Geometry: final body of the model. Coordinates: model frame, mm. Face numbers are marked on the shaded views. A direction names the side the tool comes from. Give positions to 0.01 mm unless a question says otherwise; leave off trailing zeros. Write each loop counter-clockwise with the first axis right and the second up, starting at its lowest first coordinate (ties: lowest second). Pieces come first, ordered by that corner, then holes.
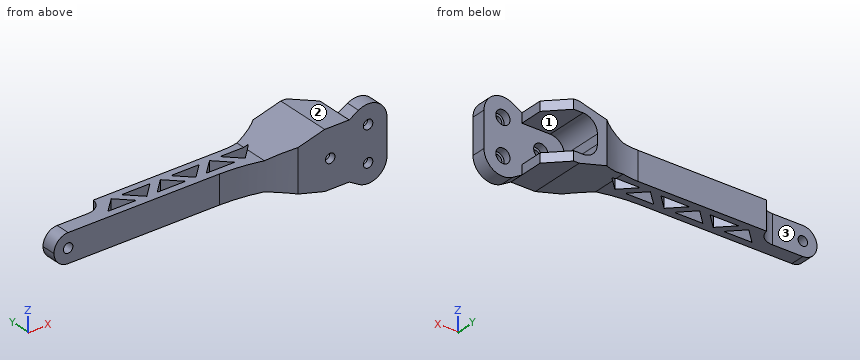
from build123d import *

# Parameters (mm, degrees)
BOSS_EXTRUDE1_DEPTH                     = 15
BOSS_EXTRUDE1_DEPTH_BACK                = 15
FILLET1_R                               = 15
BOSS_EXTRUDE2_DEPTH                     = 60
CUT_EXTRUDE5_DEPTH                      = 43
CUT_EXTRUDE5_DEPTH_BACK                 = 43
SKETCH1_6_OUTSIDE_W                     = 364.354
SKETCH1_6_OUTSIDE_H                     = 124.354
BOSS_EXTRUDE3_DEPTH                     = 15
CUT_EXTRUDE7_DEPTH                      = 256.415087263
CBORE_FOR_M5_HEX_HEAD_BOLT1_D           = 10
CBORE_FOR_M5_HEX_HEAD_BOLT1_DEPTH       = 20
CBORE_FOR_M5_HEX_HEAD_BOLT1_CBORE_D     = 15
CBORE_FOR_M5_HEX_HEAD_BOLT1_CBORE_DEPTH = 8
CBORE_FOR_M5_HEX_HEAD_BOLT1_TIP         = 3.004303095
F_10_0MM_DOWEL_HOLE1_D                  = 10
CUT_EXTRUDE9_DEPTH                      = 259.016066246
CUT_EXTRUDE14_DEPTH                     = 259.016066246


with BuildPart() as part:
    # Sketch1 → Boss-Extrude1 (new, two sides: drawn at the far end of the back side and taken through both)
    with BuildSketch(Plane.XY.offset(-BOSS_EXTRUDE1_DEPTH_BACK)):
        with BuildLine():
            Line((0, 0), (-91.545543809, 0))
            Line((-91.545543809, 0), (-91.545543809, 15))
            Line((-91.545543809, 15), (-44.293783158, 15))
            ThreePointArc((-44.293783158, 15), (-32.674833119, 19.252272915), (-26.545543809, 30))
            Line((-26.545543809, 30), (109.126292876, 30))
            ThreePointArc((109.126292876, 30), (132.446309196, 33.71762603), (153.454456191, 44.501950965))
            Line((153.454456191, 44.501950965), (188.454456191, 44.501950965))
            Line((188.454456191, 44.501950965), (208.454456191, 24.501950965))
            Line((208.454456191, 24.501950965), (208.454456191, 0))
            Line((208.454456191, 0), (208.454456191, -15.498049035))
            Line((208.454456191, -15.498049035), (154.553796185, -15.498049035))
            ThreePointArc((154.553796185, -15.498049035), (119.809900794, -3.919403897), (83.397793421, 0))
            Line((83.397793421, 0), (0, 0))
        make_face()
    extrude(amount=BOSS_EXTRUDE1_DEPTH + BOSS_EXTRUDE1_DEPTH_BACK)

    # Fillet1
    fillet1_edges = [part.edges().sort_by_distance(p)[0] for p in [
        (-91.545543809, 7.5, 15),
        (-91.545543809, 7.5, -15),
    ]]
    fillet(fillet1_edges, radius=FILLET1_R - 0.0001)  # a hair under: the kernel refuses the full size

    # Sketch2 → Boss-Extrude2 (add)
    with BuildSketch(Plane.XZ.offset(15.498049035)):
        Polygon((126.618755864, -15), (153.454456191, -22.190604231), (182.599517977, -30), (208.454456191, -30), (208.454456191, 30), (182.599517977, 30), (153.454456191, 22.190604231), (126.618755864, 15), align=None)
    extrude(amount=-BOSS_EXTRUDE2_DEPTH)

    # Sketch1<6> outside → Cut-Extrude5 (cut, two sides: drawn at the far end of the back side and taken through both)
    with BuildSketch(Plane.XY.offset(-CUT_EXTRUDE5_DEPTH_BACK)):
        with Locations((58.454, 14.502)):
            Rectangle(SKETCH1_6_OUTSIDE_W, SKETCH1_6_OUTSIDE_H)
        with BuildLine():
            Line((0, 0), (-91.545543809, 0))
            Line((-91.545543809, 0), (-91.545543809, 15))
            Line((-91.545543809, 15), (-44.293783158, 15))
            ThreePointArc((-44.293783158, 15), (-32.674833119, 19.252272915), (-26.545543809, 30))
            Line((-26.545543809, 30), (109.126292876, 30))
            ThreePointArc((109.126292876, 30), (132.446309196, 33.71762603), (153.454456191, 44.501950965))
            Line((153.454456191, 44.501950965), (188.454456191, 44.501950965))
            Line((188.454456191, 44.501950965), (208.454456191, 24.501950965))
            Line((208.454456191, 24.501950965), (208.454456191, 0))
            Line((208.454456191, 0), (208.454456191, -15.498049035))
            Line((208.454456191, -15.498049035), (154.553796185, -15.498049035))
            ThreePointArc((154.553796185, -15.498049035), (119.809900794, -3.919403897), (83.397793421, 0))
            Line((83.397793421, 0), (0, 0))
        make_face(mode=Mode.SUBTRACT)
    extrude(amount=CUT_EXTRUDE5_DEPTH + CUT_EXTRUDE5_DEPTH_BACK, mode=Mode.SUBTRACT)

    # Sketch3 → Boss-Extrude3 (add)
    with BuildSketch(Plane.XZ.offset(15.498049035)):
        with BuildLine():
            Line((208.454456191, -30), (218.39339466, -35.78511038))
            ThreePointArc((218.39339466, -35.78511038), (238.423878677, -35.838126061), (248.454456191, -18.5))
            Line((248.454456191, -18.5), (248.454456191, 18.5))
            ThreePointArc((248.454456191, 18.5), (238.423878677, 35.838126061), (218.39339466, 35.78511038))
            Line((218.39339466, 35.78511038), (208.454456191, 30))
            Line((208.454456191, 30), (208.454456191, -30))
        make_face()
    extrude(amount=-BOSS_EXTRUDE3_DEPTH)

    # Sketch4 → Cut-Extrude7 (cut, through all)
    with BuildSketch(Plane(origin=(0, -0.498049035, 0), x_dir=(1, 0, 0), z_dir=(0, 1, 0))):
        with BuildLine():
            Line((208.454456191, 20), (178.454456191, 20))
            ThreePointArc((178.454456191, 20), (167.847854474, 15.606601718), (163.454456191, 5))
            Line((163.454456191, 5), (163.454456191, -5))
            ThreePointArc((163.454456191, -5), (167.847854474, -15.606601718), (178.454456191, -20))
            Line((178.454456191, -20), (208.454456191, -20))
            Line((208.454456191, -20), (208.454456191, 20))
        make_face()
    extrude(amount=CUT_EXTRUDE7_DEPTH, mode=Mode.SUBTRACT)

    # CBORE for M5 Hex Head Bolt1
    with Locations(Plane(origin=(0, -0.498049035, 0), x_dir=(1, 0, 0), z_dir=(0, 1, 0))):
        with Locations((188.454456191, 0), (228.454456191, 18.5), (228.454456191, -18.5)):
            CounterBoreHole(CBORE_FOR_M5_HEX_HEAD_BOLT1_D / 2, CBORE_FOR_M5_HEX_HEAD_BOLT1_CBORE_D / 2, CBORE_FOR_M5_HEX_HEAD_BOLT1_CBORE_DEPTH, depth=CBORE_FOR_M5_HEX_HEAD_BOLT1_DEPTH)
            with Locations((0, 0, -(CBORE_FOR_M5_HEX_HEAD_BOLT1_DEPTH + CBORE_FOR_M5_HEX_HEAD_BOLT1_TIP / 2))):  # 118° drill point
                Cone(0, CBORE_FOR_M5_HEX_HEAD_BOLT1_D / 2, CBORE_FOR_M5_HEX_HEAD_BOLT1_TIP, mode=Mode.SUBTRACT)

    # Ø10.0mm Dowel Hole1 (through all)
    with Locations(Plane(origin=(0, 15, 0), x_dir=(1, 0, 0), z_dir=(0, 1, 0))):
        with Locations((-76.545543809, 0)):
            Hole(F_10_0MM_DOWEL_HOLE1_D / 2)

    # Sketch14 → Cut-Extrude9 (cut, through all)
    with BuildSketch(Plane.XY.offset(15)):
        Polygon((-28.545543809, 7.687067678), (-13.545543809, 22.704940786), (1.454456191, 7.687067678), align=None)
        Polygon((12.454456191, 7.687067678), (-2.545543809, 22.704940786), (27.454456191, 22.704940786), align=None)
        Polygon((49.454456191, 22.704940786), (79.454456191, 22.704940786), (64.454456191, 7.687067678), align=None)
        Polygon((23.454456191, 7.687067678), (38.454456191, 22.704940786), (53.454456191, 7.687067678), align=None)
        Polygon((75.454456191, 7.687067678), (90.454456191, 22.704940786), (105.454456191, 7.687067678), align=None)
        Polygon((116.454456191, 7.687067678), (101.454456191, 22.704940786), (131.454456191, 22.704940786), align=None)
    extrude(amount=-CUT_EXTRUDE9_DEPTH, mode=Mode.SUBTRACT)

    # Sketch14<3> → Cut-Extrude14 (cut, through all)
    with BuildSketch(Plane.XY.offset(15)):
        Polygon((116.454456191, 7.687067678), (101.454456191, 22.704940786), (131.454456191, 22.704940786), align=None)
    extrude(amount=CUT_EXTRUDE14_DEPTH, mode=Mode.SUBTRACT)


solid = part.part
Q1. Section B-B on x = 6. Output: boundary loops of the cut face in (y, z).
Filled sheet:
outline: (0, -15) - (14.15, -15) - (14.15, 15) - (0, 15) - close; (22.7, -15) - (30, -15) - (30, 15) - (22.7, 15) - close
Q2. Access query for the marked faces 1, 2 and 3. Directions: +Z, -Z, +X, -X, +Y, -Y. A direction counts if a zero-diameter tool reaches every point of the face in a straight line with its end or side. Return the directions, or none.
Filled sheet:
face 1: +X, +Y
face 2: +Z, -X, +Y, -Y
face 3: +Z, -Z, -X, +Y
Q3. Section A-A on x = 44. Output: boundary loops of the cut face in (y, z), plus the area to 3 significant figures.
Filled sheet:
outline: (0, -15) - (7.69, -15) - (7.69, 15) - (0, 15) - close; (17.15, -15) - (30, -15) - (30, 15) - (17.15, 15) - close
area: 616 mm2
Q4. Ray query, line 1 along Z through (x, y) = (223, -2.5); line 2 along Y through (x, z) = (39, 10); line 3 along Y through (x, z) = (183.5, 19). Return the intervals inside material, ascending.
Filled sheet:
line 1: z = -37.74 to -23.65, -13.35 to 13.35, 23.65 to 37.74
line 2: y = 0 to 7.69, 22.16 to 30
line 3: y = -15.5 to -0.5
Q5. Pin query (flat end, axial travel): P1, Ø9, axis at x = 228.45, z = 18.5, coming from the -Y side; P2, Ø9, axis at x = -75.5, z = -3, coming from the +Y side; P3, Ø19.5, axis at x = 228.45, z = -18.5, coming from the +Y side; P4, Ø13.5, axis at x = 188.45, z = 0, coming from the -Y side. Return the tip coordinate at first contact, or that it passes through.
Filled sheet:
P1: passes through
P2: stops at y = 15
P3: stops at y = -0.5
P4: stops at y = -15.5
